CAD build for the part. Positions are in the model's coordinates, mm. Face numbers are marked on the shaded views. A direction names the side the tool comes from. Coordinates: 2 decimals unless noted, no trailing zeros. Order: outer loops, then holes, each group sorted by start corner. A loop starts at its lowest first (then second) coordinate and runs counter-clockwise, first axis right, second up. Notation, with made-up numbers: (-10, -23.5) -> (36, -23.5) arc R23 cw to (36, 3.5) -> close; hole circle Ø9 at (70.5, 75). An arc over 180 degrees is marked (long way). Use one line per item in the form item = value. Start each with the question number.
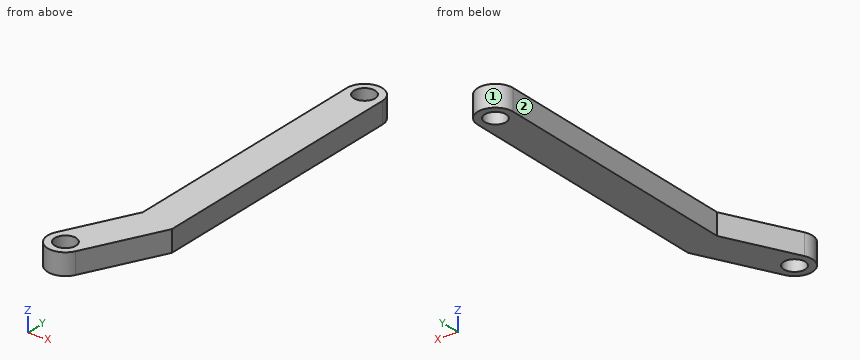
from build123d import *

# Parameters (mm, degrees)
SKETCH1_R           = 15
BOSS_EXTRUDE1_DEPTH = 30


with BuildPart() as part:
    # Sketch1 → Boss-Extrude1 (new body)
    with BuildSketch(Plane.XY):
        with BuildLine():
            Line((-61.054066009, 459.688422397), (-61.054066009, 88.319905145))
            Line((-61.054066009, 88.319905145), (-108.868464608, -8.595458486))
            ThreePointArc((-108.868464608, -8.595458486), (-97.509706692, -42.076477267), (-64.028687911, -30.717719351))
            Line((-64.028687911, -30.717719351), (-11.054066009, 76.656939649))
            Line((-11.054066009, 76.656939649), (-11.054066009, 459.688422397))
            ThreePointArc((-11.054066009, 459.688422397), (-36.054066009, 484.688422397), (-61.054066009, 459.688422397))
        make_face()
        with Locations((-36.054066009, 459.688422397)):
            Circle(SKETCH1_R, mode=Mode.SUBTRACT)
        with Locations((-86.44857626, -19.656588918)):
            Circle(SKETCH1_R, mode=Mode.SUBTRACT)
    extrude(amount=BOSS_EXTRUDE1_DEPTH)


solid = part.part
1) Cut at D-D on x = -26. Give the cut face in (y, z).
2) 3-axis set-ups, long thin cutter, end or side, ignore diameter. For the marked faces 1 and 2: which of +Z, -Z, +X, -X, +Y, -Y reach the whole face in a straight line?
3) Drop flat-ended pins along their axis: P1, Ø12, axis at y = 80, z = 21, coming from the -X side; P2, Ø12, axis at x = -83, z = 4.5, coming from the +Y side; P3, Ø3, axis at x = -84.5, z = 26, coming from the -Y side. Give the stop position or say it passes through.
4) Cut at A-A on z = 23.5. Give the cut face in (x, y).
5) Cut at B-B on x = -95. Give the cut face in (y, z).
6) Cut at C-C on y = 165. Give the cut face in (x, z), then the cut area to 3 significant figures.
7) Probe L1, parallel to X at y = 373, z = 6.75; L2, parallel to Y at x = -45, z = 16.5; L3, parallel to X at y = -8, z = 18. List the from-to ranges inside material, lowest first.
Values follow:
q1.outline = (46.36, 0) -> (448.56, 0) -> (448.56, 30) -> (46.36, 30) -> close; (470.82, 0) -> (482.58, 0) -> (482.58, 30) -> (470.82, 30) -> close
q2.face_1 = +Z, -Z, +Y
q2.face_2 = +Z, -Z, -X, +Y
q3.P1 = -68.12
q3.P2 = 56
q3.P3 = -44.65
q4.outline = (-108.87, -8.6) arc R25 ccw to (-64.03, -30.72) -> (-11.05, 76.66) -> (-11.05, 459.69) arc R25 ccw to (-61.05, 459.69) -> (-61.05, 88.32) -> close; hole circle Ø30 at (-86.45, -19.66); hole circle Ø30 at (-36.05, 459.69)
q5.outline = (-43.15, 0) -> (-31.98, 0) -> (-31.98, 30) -> (-43.15, 30) -> close; (-7.33, 0) -> (19.51, 0) -> (19.51, 30) -> (-7.33, 30) -> close
q6.outline = (-61.05, 0) -> (-11.05, 0) -> (-11.05, 30) -> (-61.05, 30) -> close
q6.area = 1,500 mm^2
q7.L1 = -61.05 to -11.05
q7.L2 = 7.85 to 447.65, 471.73 to 483.03
q7.L3 = -108.57 to -95.89, -77.01 to -52.82
